Input: part model. Units: mm. Frame: model coordinates. Face numbers are marked on the shaded views. A direction names the side the tool comes from. Round coordinates to 2 decimals unless told otherwise and drop trailing zeros. Loops run counter-clockwise (first coordinate to the right, second up) from the corner with the lowest first, then second, coordinate; pieces in that order, holes last. Notation, with made-up numbers: (62.5, -1) -> (67.5, -1) arc R19 cw to (67.5, 12) -> close; hole circle Ø10 at (-16, -19.75). An arc over 180 degrees is marked (long way). Answer as a JSON object with one key per item and string values. Group by question number.
Item 1: Pin query (flat end, axial travel): pin 1 (4 mm diameter, centred on x = 63, z = 15, fed in from -Y); pin 2 (1.9 mm diameter, centred on x = 50.5, z = -20.5, fed in from +Y); pin 3 (1.9 mm diameter, centred on y = -78.5, z = -19, fed in from +X); pin 4 (5 mm diameter, centred on x = 50.8, y = -147.95, fed in from -Z). Return the tip coordinate at first contact, or that it passes through.
Item 2: Material intervals for line 1 (Y direction, x = 73, z = -9); line 2 (X direction, y = -15.5, z = -2); line 3 (Y direction, x = 50.8, z = -19), sorted ascending. Write a range as [from, to].
Item 3: Section query D-D on y = -108.5. Return loops of the section in (x, z), and give its area (3 significant figures).
Item 4: Draft query along Y for the marked faces 4, 5, 6 and 7. Return one class per face: released by +Y, released by -Y, zero draft, split by the parting line, or undercut.
Item 5: Set-up query: the marked faces 1, 2 and 3. Return all of +Z, -Z, +X, -X, +Y, -Y with unobstructed straight access to the full face (end or side cutting, diameter ignored); none if empty.
Item 6: Section query C-C on y = 57. Return loops of the section in (x, z), and give its area (3 significant figures).
Item 7: Section query B-B on x = 18.5. Return loops of the section in (y, z), and give its area (3 significant figures).
Item 8: Section query A-A on z = 2.5. Return loops of the section in (x, y), and give its area (3 significant figures).
from build123d import *

# Parameters (mm, degrees)
F0_W      = 152.4
F0_H      = 38.1
F1_DEPTH  = 101.6
F2_W      = 88.9
F2_H      = 139.7
F3_DEPTH  = 31.75
F4_R      = 6.35
F5_DEPTH  = 101.6
F6_W      = 12.7
F6_H      = 20.32
F7_DEPTH  = 6.35
F8_W      = 12.7
F8_H      = 6.35
F9_DEPTH  = 76.2
F10_R     = 1.905
F11_DEPTH = 6.35
F12_R     = 5.08


# Not quite as in the source:
# - two fillets or chamfers of one size are made in one step
# - a feature names something its author has since deleted; it is built from what else it names


with BuildPart() as f1:
    # F0 (on Right) → F1 (new body)
    with BuildSketch(Plane.YZ):
        with Locations((3.7253e-06, 2.6738062448)):
            Rectangle(F0_W, F0_H)
    extrude(amount=F1_DEPTH)

    # F2 (on face) → F3 (cut)
    with BuildSketch(Plane.XY.offset(21.7238062448)):
        with Locations((50.8, 3.7253e-06)):
            Rectangle(F2_W, F2_H)
    extrude(amount=-F3_DEPTH, mode=Mode.SUBTRACT)

    # F4 (on face) → F5 (cut)
    with BuildSketch(Plane.YZ.offset(101.6)):
        with Locations((31.7500037253, -8.2481937552)):
            Circle(F4_R)
    extrude(amount=-F5_DEPTH, mode=Mode.SUBTRACT)

    # F6 (on face) → F7 (join)
    with BuildSketch(Plane(origin=(0, 0, -16.3761937552), x_dir=(1, 0, 0), z_dir=(0, 0, -1))):
        with Locations((50.8, 66.0399962747)):
            Rectangle(F6_W, F6_H)
    extrude(amount=F7_DEPTH)

    # F8 (on face) → F9 (join)
    with BuildSketch(Plane.XZ.offset(76.1999962747)):
        with Locations((50.8, -19.5511937552)):
            Rectangle(F8_W, F8_H)
    extrude(amount=F9_DEPTH)

    # F10 (on face) → F11 (cut)
    with BuildSketch(Plane.XY.offset(-16.3761937552)):
        with Locations((50.8, -147.9549962747)):
            Circle(F10_R)
    extrude(amount=-F11_DEPTH, mode=Mode.SUBTRACT)

    # F12
    f12_edges = [f1.edges().sort_by_distance(p)[0] for p in [
        (44.45, -152.399996, -19.551194),
        (57.15, -152.399996, -19.551194),
    ]]
    fillet(f12_edges, radius=F12_R)


solid = f1.part
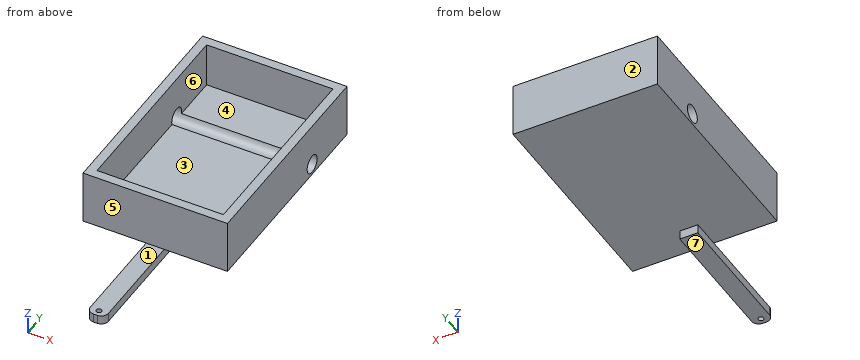
Solved:
{
 "1": {"pin 1": "y = -76.2", "pin 2": "y = -55.88", "pin 3": "x = 57.15", "pin 4": "z = -22.73"},
 "2": {"line 1": "[-76.2, -69.85], [69.85, 76.2]", "line 2": "[0, 6.35], [95.25, 101.6]", "line 3": "[-152.4, -149.86], [-146.05, -55.88]"},
 "3": {"outline": "(44.45, -22.73) -> (57.15, -22.73) -> (57.15, -16.38) -> (44.45, -16.38) -> close", "area": "80.6 mm²"},
 "4": {"face 4": "undercut", "face 5": "released by -Y", "face 6": "undercut", "face 7": "zero draft"},
 "5": {"face 1": "+Z, +X, -X, -Y", "face 2": "+Z, -Z, +X, -X, +Y", "face 3": "+Z"},
 "6": {"outline": "(0, -16.38) -> (101.6, -16.38) -> (101.6, 21.72) -> (95.25, 21.72) -> (95.25, -10.03) -> (6.35, -10.03) -> (6.35, 21.72) -> (0, 21.72) -> close", "area": "1,050 mm²"},
 "7": {"outline": "(-76.2, -16.38) -> (76.2, -16.38) -> (76.2, 21.72) -> (69.85, 21.72) -> (69.85, -10.03) -> (37.85, -10.03) arc R6.35 cw to (25.65, -10.03) -> (-69.85, -10.03) -> (-69.85, 21.72) -> (-76.2, 21.72) -> close", "area": "1,330 mm²"},
 "8": {"outline": "(0, -76.2) -> (101.6, -76.2) -> (101.6, 76.2) -> (0, 76.2) -> close; hole (6.35, -69.85) -> (95.25, -69.85) -> (95.25, 69.85) -> (6.35, 69.85) -> close", "area": "3,060 mm²"}
}
